```python
from build123d import *

# Parameters (mm, degrees)
SKETCH1_R           = 30
BOSS_EXTRUDE1_DEPTH = 5
SKETCH2_R           = 1.25
CUT_EXTRUDE1_DEPTH  = 5
SKETCH3_R           = 2.5
BOSS_EXTRUDE2_DEPTH = 25
BOSS_EXTRUDE3_START = 60
SKETCH4_R           = 2.5
BOSS_EXTRUDE3_DEPTH = 60


with BuildPart() as part:
    # Sketch1 → Boss-Extrude1 (new body)
    with BuildSketch(Plane.XY):
        Circle(SKETCH1_R)
    extrude(amount=BOSS_EXTRUDE1_DEPTH)

    # Sketch2 → Cut-Extrude1 (cut)
    with BuildSketch(Plane.XY.offset(5)):
        with Locations((0, 15.5)):
            Circle(SKETCH2_R)
        with Locations((15.5, 0)):
            Circle(SKETCH2_R)
        with Locations((0, -15.5)):
            Circle(SKETCH2_R)
        with Locations((-15.5, 0)):
            Circle(SKETCH2_R)
        with Locations((4.242640687, 4.242640687)):
            Circle(SKETCH2_R)
        with Locations((4.242640687, -4.242640687)):
            Circle(SKETCH2_R)
        with Locations((-4.242640687, -4.242640687)):
            Circle(SKETCH2_R)
        with Locations((-4.242640687, 4.242640687)):
            Circle(SKETCH2_R)
    extrude(amount=-CUT_EXTRUDE1_DEPTH, mode=Mode.SUBTRACT)

    # Sketch3 → Boss-Extrude2 (add)
    with BuildSketch(Plane(origin=(0, 0, 0), x_dir=(-1, 0, 0), z_dir=(0, 0, -1))):
        with Locations(Location((0, 0, 0), (0, 0, 180))):
            Circle(SKETCH3_R)
    extrude(amount=BOSS_EXTRUDE2_DEPTH)

    # Sketch4 → Boss-Extrude3 (add)
    with BuildSketch(Plane.XY.offset(5).offset(BOSS_EXTRUDE3_START)):
        Circle(SKETCH4_R)
    extrude(amount=-BOSS_EXTRUDE3_DEPTH)


solid = part.part
```
Verification items for the finished model (mm, model axes). A direction names the side the tool comes from. Coordinates: 2 decimals unless noted, no trailing zeros. Loops run counter-clockwise (first coordinate to the right, second up) from the corner with the lowest first, then second, coordinate; pieces in that order, holes last. Notation, with made-up numbers: (26, 50) -> (80, 50) arc R13 cw to (80, 72) -> close; hole circle Ø2 at (75, 5.5). An arc over 180 degrees is marked (long way). Answer in a Markdown table with one row per item. Add a question column.
1. Material ranges on probe 1 along Y at (x, z) = (0, 2); probe 2 along Z at (x, y) = (13, -22.5); probe 3 along X at (y, z) = (1, 34), recorded low to high. Write a range as [from, to].
2. Section check A-A, the plane y = 0. Enter the section's corners in (x, z), then the cut area to 3 significant figures.
3. Draft check along Y on faces 3 (the face through (5.4, -4.72, 2.54)), 4 (the face through (-5.49, -4.19, 2.54)), 5 (the face through (6, 0, 5)), 6 (the face through (-2.5, -0.1, -12.3)). Enter one of: +Y half, -Y half, draft (parallel to the pull), parting line (faces both ways), or undercut.
4. Section check C-C, the plane y = 15.5. Enter the section's corners in (x, z).
5. Access from +Z, -Z, +X, -X, +Y, -Y to the whole of each face (thin tool, end or side, straight path). Record for faces 1 (the face through (-29.97, 1.32, 2.46)), 2 (the face through (-0.54, -2.44, 35.42)).
6. Depth check by flat-ended pin: P1, Ø3, axis at x = -13.5, y = -6, coming from the -Z side; P2, Ø1, axis at x = 15, y = -22, coming from the +Z side; P3, Ø2, axis at x = -1, z = 44, coming from the -Y side. Enter the tip coordinate at first touch or a pass-through.
Derived:
| question | item | result |
|---|---|---|
| 1 | probe 1 | y = [-30, -16.75], [-14.25, 14.25], [16.75, 30] |
| 1 | probe 2 | z = [0, 5] |
| 1 | probe 3 | x = [-2.29, 2.29] |
| 2 | outline | (-30, 0) -> (-16.75, 0) -> (-16.75, 5) -> (-30, 5) -> close; (-14.25, 0) -> (-2.5, 0) -> (-2.5, -25) -> (2.5, -25) -> (2.5, 0) -> (14.25, 0) -> (14.25, 5) -> (2.5, 5) -> (2.5, 65) -> (-2.5, 65) -> (-2.5, 5) -> (-14.25, 5) -> close; (16.75, 0) -> (30, 0) -> (30, 5) -> (16.75, 5) -> close |
| 2 | area | 700 mm² |
| 3 | face 3 | undercut |
| 3 | face 4 | undercut |
| 3 | face 5 | draft |
| 3 | face 6 | parting line |
| 4 | outline | (-25.69, 0) -> (-1.25, 0) -> (-1.25, 5) -> (-25.69, 5) -> close; (1.25, 0) -> (25.69, 0) -> (25.69, 5) -> (1.25, 5) -> close |
| 5 | face 1 | +Z, -Z |
| 5 | face 2 | +Z |
| 6 | P1 | stops at z = 0 |
| 6 | P2 | stops at z = 5 |
| 6 | P3 | stops at y = -2.5 |
